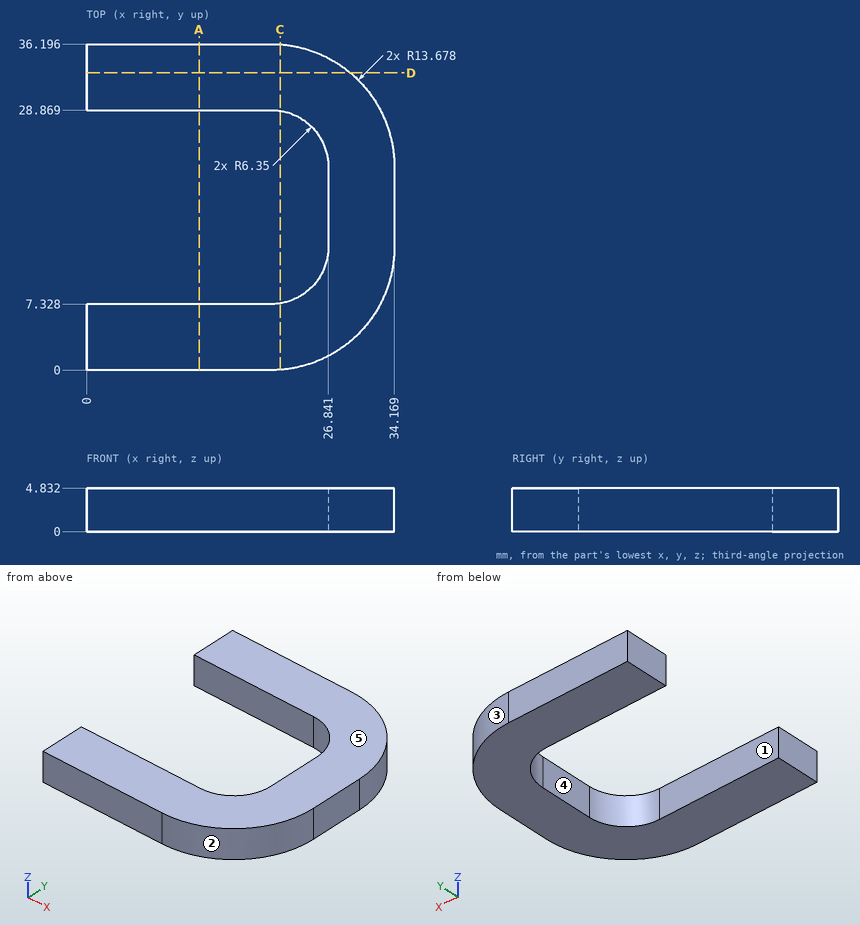
Geometry check sheet. Reference: drawing and pictorial views, mm from the part's lowest x, y, z. A direction names the side the tool comes from. Round coordinates to 2 decimals unless told otherwise and drop trailing zeros. Order: outer loops, then holes, each group sorted by start corner. A loop starts at its lowest first (then second) coordinate and runs counter-clockwise, first axis right, second up. Notation, with made-up numbers: M 21.5,-34.75 L 31.5,-34.75 A16 cw 31.5,-7.75 Z; hole C 77.5,58 d11. An arc over 180 degrees is marked long. Write item = value, one per line.
Q1. Section check A-A (x = 12.5). Enter the section's corners in (y, z).
Answer block:
outline = M 0,0 L 7.33,0 L 7.33,4.83 L 0,4.83 Z; M 28.87,0 L 36.2,0 L 36.2,4.83 L 28.87,4.83 Z
Q2. Section check C-C (x = 21.5). Enter the section's corners in (y, z).
Answer block:
outline = M 0.04,0 L 7.41,0 L 7.41,4.83 L 0.04,4.83 Z; M 28.79,0 L 36.16,0 L 36.16,4.83 L 28.79,4.83 Z
Q3. Scan lines: line 1 (Y direction, x = 18, z = 4.3); line 2 (X direction, y = 13.5, z = 2.15); line 3 (X direction, y = 7, z = 2.15). Record each from-to range of solid material in increasing order.
Answer block:
line_1 = 0 to 7.33, 28.87 to 36.2
line_2 = 26.84 to 34.17
line_3 = 0 to 32.43
Q4. Depth check by flat-ended pin: pin 1 Ø2 at (y, z) = (19, 1.5) entering from -X; pin 2 Ø1.5 at (y, z) = (6, 1) entering from +X (1 decimal). Enter the tip coordinate at first touch or a pass-through.
Answer block:
pin_1 = 26.84
pin_2 = 32.3
Q5. Release check for a two-part mould opening along Y. For the marked faces 1, 2 and 3 record: released by +Y, released by -Y, zero draft, split by the parting line, or undercut.
Answer block:
face_1 = undercut
face_2 = released by -Y
face_3 = released by +Y
Q6. Section check D-D (y = 33). Enter the section's corners in (x, z).
Answer block:
outline = M 0,0 L 29.28,0 L 29.28,4.83 L 0,4.83 Z
Q7. Set-up check for the marked faces 4 and 5: record each of +Z, -Z, +X, -X, +Y, -Y from which the full face is reachable in a straight line by a thin tool's end or side.
Answer block:
face_4 = +Z, -Z, -X
face_5 = +Z, +X, -X, +Y, -Y
